CAD build for the part. Positions are in the model's coordinates, mm. A direction names the side the tool comes from. Round coordinates to 2 decimals unless told otherwise and drop trailing zeros. Loops run counter-clockwise (first coordinate to the right, second up) from the corner with the lowest first, then second, coordinate; pieces in that order, holes last.
```python
from build123d import *

# Parameters (mm, degrees)
SKETCH_1_W          = 40
SKETCH_1_H          = 50
SKETCH_1_R          = 1.6
EXTRUDE_1_DEPTH     = 3
SKETCH_2_W          = 8
SKETCH_2_H          = 3
EXTRUDE_2_DEPTH     = 15
SKETCH_3_W          = 40
SKETCH_3_H          = 56
EXTRUDE_3_DEPTH     = 3
CUT_EXTRUDE_1_REACH = 40.833
SKETCH_4_W          = 40
SKETCH_4_H          = 32
CUT_EXTRUDE_START   = -3
SKETCH_5_W          = 24
SKETCH_5_H          = 50
CUT_EXTRUDE_2_DEPTH = 3
FILLET_1_R          = 1
CUT_EXTRUDE_4_REACH = 39.537
SKETCH_10_W         = 20
SKETCH_10_H         = 30
SKETCH_11_W         = 3
SKETCH_11_H         = 18
EXTRUDE_4_DEPTH     = 10
CUT_EXTRUDE_5_REACH = 58.009
SKETCH_12_R         = 1.6
FILLET_2_R          = 1


with BuildPart() as part:
    # 草图1 → 凸台-拉伸1 (new body)
    with BuildSketch(Plane.XY):
        Rectangle(SKETCH_1_W, SKETCH_1_H)
        with Locations((-15, 20)):
            Circle(SKETCH_1_R, mode=Mode.SUBTRACT)
        with Locations((15, 20)):
            Circle(SKETCH_1_R, mode=Mode.SUBTRACT)
        with Locations((15, -20)):
            Circle(SKETCH_1_R, mode=Mode.SUBTRACT)
        with Locations((-15, -20)):
            Circle(SKETCH_1_R, mode=Mode.SUBTRACT)
    extrude(amount=EXTRUDE_1_DEPTH)

    # 草图2 → 凸台-拉伸2 (add)
    with BuildSketch(Plane(origin=(0, 0, 0), x_dir=(-1, 0, 0), z_dir=(0, 0, -1))):
        with Locations((-16, 26.5)):
            Rectangle(SKETCH_2_W, SKETCH_2_H)
        with Locations((16, 26.5)):
            Rectangle(SKETCH_2_W, SKETCH_2_H)
        with Locations((-16, -26.5)):
            Rectangle(SKETCH_2_W, SKETCH_2_H)
        with Locations((16, -26.5)):
            Rectangle(SKETCH_2_W, SKETCH_2_H)
    extrude(amount=-EXTRUDE_2_DEPTH)

    # 草图3 → 凸台-拉伸3 (add)
    with BuildSketch(Plane.XY.offset(15)):
        Rectangle(SKETCH_3_W, SKETCH_3_H)
    extrude(amount=EXTRUDE_3_DEPTH)

    # 草图4 → 切除-拉伸1 (cut, up to next)
    with BuildSketch(Plane(origin=(0, 0, 0), x_dir=(-1, 0, 0), z_dir=(0, 0, -1)), mode=Mode.PRIVATE) as cut_extrude_1_sk1:
        Rectangle(SKETCH_4_W, SKETCH_4_H)
    cut_extrude_1_tool1 = extrude(cut_extrude_1_sk1.sketch, amount=-CUT_EXTRUDE_1_REACH, mode=Mode.PRIVATE) & part.part
    add(cut_extrude_1_tool1.solids().sort_by_distance((0, 0, 0))[0], mode=Mode.SUBTRACT)

    # 草图5 → 切除-拉伸2 (cut)
    with BuildSketch(Plane(origin=(0, 0, 0), x_dir=(-1, 0, 0), z_dir=(0, 0, -1)).offset(CUT_EXTRUDE_START)):
        Rectangle(SKETCH_5_W, SKETCH_5_H)
    extrude(amount=CUT_EXTRUDE_2_DEPTH, mode=Mode.SUBTRACT)

    # 圆角1
    fillet_1_edges = [part.edges().sort_by_distance(p)[0] for p in [
        (20, -16, 1.5),
        (20, 16, 1.5),
        (12, 16, 1.5),
        (-12, 16, 1.5),
        (12, -16, 1.5),
        (-12, -16, 1.5),
    ]]
    fillet(fillet_1_edges, radius=FILLET_1_R)

    # 草图10 → 切除-拉伸4 (cut, up to next)
    with BuildSketch(Plane(origin=(0, 0, 15), x_dir=(-1, 0, 0), z_dir=(0, 0, -1)), mode=Mode.PRIVATE) as cut_extrude_4_sk1:
        Rectangle(SKETCH_10_W, SKETCH_10_H)
    cut_extrude_4_tool1 = extrude(cut_extrude_4_sk1.sketch, amount=-CUT_EXTRUDE_4_REACH, mode=Mode.PRIVATE) & part.part
    add(cut_extrude_4_tool1.solids().sort_by_distance((0, 0, 15))[0], mode=Mode.SUBTRACT)

    # 草图11 → 凸台-拉伸4 (add)
    with BuildSketch(Plane(origin=(0, 28, 0), x_dir=(1, 0, 0), z_dir=(0, 1, 0))):
        with Locations((-18.5, -9)):
            Rectangle(SKETCH_11_W, SKETCH_11_H)
    extrude_4 = extrude(amount=EXTRUDE_4_DEPTH)

    # 镜向1: 凸台-拉伸4 across plane
    add(extrude_4.mirror(Plane.ZX))

    # 草图12 → 切除-拉伸5 (cut, up to next)
    with BuildSketch(Plane(origin=(-17, 0, 0), x_dir=(0, 0, -1), z_dir=(1, 0, 0)), mode=Mode.PRIVATE) as cut_extrude_5_sk1:
        with Locations((-9, 32.75)):
            Circle(SKETCH_12_R)
    cut_extrude_5_tool1 = extrude(cut_extrude_5_sk1.sketch, amount=-CUT_EXTRUDE_5_REACH, mode=Mode.PRIVATE) & part.part
    # 草图12 → 切除-拉伸5 (cut, up to next)
    with BuildSketch(Plane(origin=(-17, 0, 0), x_dir=(0, 0, -1), z_dir=(1, 0, 0)), mode=Mode.PRIVATE) as cut_extrude_5_sk2:
        with Locations((-9, -32.75)):
            Circle(SKETCH_12_R)
    cut_extrude_5_tool2 = extrude(cut_extrude_5_sk2.sketch, amount=-CUT_EXTRUDE_5_REACH, mode=Mode.PRIVATE) & part.part
    add(cut_extrude_5_tool1.solids().sort_by_distance((-17, 32.75, 9))[0], mode=Mode.SUBTRACT)
    add(cut_extrude_5_tool2.solids().sort_by_distance((-17, -32.75, 9))[0], mode=Mode.SUBTRACT)

    # 圆角2
    fillet_2_edges = [part.edges().sort_by_distance(p)[0] for p in [
        (-18.5, 38, 18),
        (-18.5, 38, 0),
        (-18.5, -38, 0),
        (-18.5, -38, 18),
    ]]
    fillet(fillet_2_edges, radius=FILLET_2_R)


solid = part.part
```
Item 1: Cut at C-C, the plane x = 2.5. Give the cut face in (y, z).
Answers follow:
outline: (-28, 15) - (-15, 15) - (-15, 18) - (-28, 18) - close; (15, 15) - (28, 15) - (28, 18) - (15, 18) - close
Item 2: 3-axis set-ups, long thin cutter, end or side, ignore diameter. For faces 5 (the flat face through (-16, 16, 1)), 6 (the flat face through (-10, 0, 16)), 7 (the flat face through (16, 25, 9)), 8 (the flat face through (5, -28, 17)): which of +Z, -Z, +X, -X, +Y, -Y reach the whole face in a straight line?
Answers follow:
face 5: -Z, +X, -X
face 6: +Z, -Z
face 7: +X, -X
face 8: +Z, -Z, +X, -Y
Item 3: Cut at A-A, the plane y = 9. Give the cut face in (x, z).
Answers follow:
outline: (-20, 15) - (-10, 15) - (-10, 18) - (-20, 18) - close; (10, 15) - (20, 15) - (20, 18) - (10, 18) - close
Item 4: Two-plate mould, pull along Z, no slides. Class faces 1 (the flat face through (-16, -25, 9)), 2 (the cylindrical face through (-16.18, -18.92, 1.48)), 3 (the flat face through (16, 22, 0)), 4 (the flat face through (-17, 21, 3)): released by +Z, released by -Z, zero draft, split by the parting line, or undercut.
Answers follow:
face 1: undercut
face 2: zero draft
face 3: released by -Z
face 4: undercut
Item 5: Cut at B-B, the plane y = -22.5. Give the cut face in (x, z), plus the area to 3 significant figures.
Answers follow:
outline: (-20, 0) - (-12, 0) - (-12, 3) - (-20, 3) - close; (-20, 15) - (20, 15) - (20, 18) - (-20, 18) - close; (12, 0) - (20, 0) - (20, 3) - (12, 3) - close
area: 168 mm2
Item 6: Cut at D-D, the plane z = 13.5. Give the cut face in (x, y), plus the area to 3 significant figures.
Answers follow:
outline: (-20, -38) - (-17, -38) - (-17, -28) - (-12, -28) - (-12, -25) - (-20, -25) - close; (-20, 25) - (-12, 25) - (-12, 28) - (-17, 28) - (-17, 38) - (-20, 38) - close; (12, -28) - (20, -28) - (20, -25) - (12, -25) - close; (12, 25) - (20, 25) - (20, 28) - (12, 28) - close
area: 156 mm2
Item 7: Probe line 1 (Y direction, x = -17.8, z = 9); line 2 (Y direction, x = 15, z = 1.2); line 3 (X direction, y = 24.5, z = 2.25). List the from-to ranges inside material, lowest first.
Answers follow:
line 1: y = -38 to -34.35, -31.15 to -25, 25 to 31.15, 34.35 to 38
line 2: y = -28 to -21.6, -18.4 to -16, 16 to 18.4, 21.6 to 28
line 3: x = -20 to -12, 12 to 20
Item 8: Flat gauge pins, fed straight in: P1, Ø5, axis at x = 15, y = 20, coming from the -Z side; P2, Ø3.5, axis at x = 15, z = 1.5, coming from the +Y side; P3, Ø12, axis at x = 0, y = -15.5, coming from the -Z side; P4, Ø5, axis at x = 15.5, z = 15.5, coming from the -Y side. Where does each tip first touch, or does it go through?
Answers follow:
P1: stops at z = 0
P2: stops at y = 28
P3: stops at z = 15
P4: stops at y = -28
